from build123d import *

# Parameters (mm, degrees)
TOP_COVER_W         = 120
TOP_COVER_H         = 25
BOSS_EXTRUDE1_DEPTH = 3
ATTACHMENT_POINT_W  = 8
ATTACHMENT_POINT_H  = 15
CUT_EXTRUDE1_DEPTH  = 2
SKETCH4_R           = 1.75
M3_SCREW_CUT_DEPTH  = 62.361632964
FILLET1_R           = 2
FILLET2_R           = 2
FILLET3_R           = 2
FILLET4_R           = 2


with BuildPart() as part:
    # Top Cover → Boss-Extrude1 (new body)
    with BuildSketch(Plane(origin=(0, 0, 0), x_dir=(1, 0, 0), z_dir=(0, 1, 0))):
        Rectangle(TOP_COVER_W, TOP_COVER_H)
    extrude(amount=BOSS_EXTRUDE1_DEPTH)

    # Attachment Point → Cut-Extrude1 (cut)
    with BuildSketch(Plane(origin=(0, 3, 0), x_dir=(1, 0, 0), z_dir=(0, 1, 0))):
        with Locations((-11, 0)):
            Rectangle(ATTACHMENT_POINT_W, ATTACHMENT_POINT_H)
        with Locations((11, 0)):
            Rectangle(ATTACHMENT_POINT_W, ATTACHMENT_POINT_H)
    extrude(amount=-CUT_EXTRUDE1_DEPTH, mode=Mode.SUBTRACT)

    # Sketch4 → M3 Screw CUT (cut, through all)
    with BuildSketch(Plane(origin=(0, 3, 0), x_dir=(1, 0, 0), z_dir=(0, 1, 0))):
        with Locations(Location((-11, 0, 0), (0, 0, 270))):
            Circle(SKETCH4_R)
        with Locations(Location((11, 0, 0), (0, 0, 90))):
            Circle(SKETCH4_R)
    extrude(amount=-M3_SCREW_CUT_DEPTH, mode=Mode.SUBTRACT)

    # Fillet1
    fillet1_edges = [part.edges().sort_by_distance(p)[0] for p in [
        (-60, 1.5, 12.5),
    ]]
    fillet(fillet1_edges, radius=FILLET1_R)

    # Fillet2
    fillet2_edges = [part.edges().sort_by_distance(p)[0] for p in [
        (60, 1.5, 12.5),
    ]]
    fillet(fillet2_edges, radius=FILLET2_R)

    # Fillet3
    fillet3_edges = [part.edges().sort_by_distance(p)[0] for p in [
        (60, 1.5, -12.5),
    ]]
    fillet(fillet3_edges, radius=FILLET3_R)

    # Fillet4
    fillet4_edges = [part.edges().sort_by_distance(p)[0] for p in [
        (-60, 1.5, -12.5),
    ]]
    fillet(fillet4_edges, radius=FILLET4_R)


solid = part.part
Read the model definition and answer for the solid it produces. Units are mm, in the model's axes. A direction names the side the tool comes from. Coordinates: 2 decimals unless noted, no trailing zeros. Order: outer loops, then holes, each group sorted by start corner. A loop starts at its lowest first (then second) coordinate and runs counter-clockwise, first axis right, second up. Notation, with made-up numbers: (8, 65.5) -> (46, 65.5) arc R20 cw to (46, 100.5) -> close; hole circle Ø3 at (72.25, 30). An arc over 180 degrees is marked (long way). Answer as a JSON object with one key per item and string values.
1) A cutting plane is placed at D-D, the plane z = 5.75. Determine the outline of the cut face in (x, y).
Model answer:
{"outline": "(-60, 0) -> (60, 0) -> (60, 3) -> (15, 3) -> (15, 1) -> (7, 1) -> (7, 3) -> (-7, 3) -> (-7, 1) -> (-15, 1) -> (-15, 3) -> (-60, 3) -> close"}
2) Each of these flat-tipped pins is pushed along its axis until it touches: pin 1 (3 mm diameter, centred on x = 11, z = 0, fed in from -Y); pin 2 (3 mm diameter, centred on x = 9.5, z = 4, fed in from +Y). Where does it stop, or does it pass through?
Model answer:
{"pin 1": "passes through", "pin 2": "stops at y = 1"}
3) A cutting plane is placed at A-A, the plane x = 11. Determine the outline of the cut face in (y, z).
Model answer:
{"outline": "(0, -12.5) -> (3, -12.5) -> (3, -7.5) -> (1, -7.5) -> (1, -1.75) -> (0, -1.75) -> close; (0, 1.75) -> (1, 1.75) -> (1, 7.5) -> (3, 7.5) -> (3, 12.5) -> (0, 12.5) -> close"}
4) A cutting plane is placed at C-C, the plane y = 2. Determine the outline of the cut face in (x, z), plus the area to 3 significant figures.
Model answer:
{"outline": "(-60, -10.5) arc R2 ccw to (-58, -12.5) -> (58, -12.5) arc R2 ccw to (60, -10.5) -> (60, 10.5) arc R2 ccw to (58, 12.5) -> (-58, 12.5) arc R2 ccw to (-60, 10.5) -> close; hole (-15, -7.5) -> (-7, -7.5) -> (-7, 7.5) -> (-15, 7.5) -> close; hole (7, -7.5) -> (15, -7.5) -> (15, 7.5) -> (7, 7.5) -> close", "area": "2,760 mm²"}
5) A cutting plane is placed at B-B, the plane z = 0. Determine the outline of the cut face in (x, y).
Model answer:
{"outline": "(-60, 0) -> (-12.75, 0) -> (-12.75, 1) -> (-15, 1) -> (-15, 3) -> (-60, 3) -> close; (-9.25, 0) -> (9.25, 0) -> (9.25, 1) -> (7, 1) -> (7, 3) -> (-7, 3) -> (-7, 1) -> (-9.25, 1) -> close; (12.75, 0) -> (60, 0) -> (60, 3) -> (15, 3) -> (15, 1) -> (12.75, 1) -> close"}
6) The mould has two halves that part along X. Classify faces 1 (the face through (-60, 1, 0)), 2 (the face through (-9.265, 0.507, -0.228)), 3 (the face through (-1, 1, -12.5)): released by +X, released by -X, zero draft, split by the parting line, or undercut.
Model answer:
{"face 1": "released by -X", "face 2": "undercut", "face 3": "zero draft"}
7) A tool of negligible diameter and unlimited length cuts with its end or side. For faces 4 (the face through (59.4, 1.52, 11.93)), 5 (the face through (-11, 1, -2)), from which of +Z, -Z, +X, -X, +Y, -Y can it reach the whole face along a straight path? Write none if from no direction.
Model answer:
{"face 4": "+Z, +X, +Y, -Y", "face 5": "+Y"}
8) Consider line 1 along X through (y, z) = (2.25, -6.5); line 2 along X through (y, z) = (0.7, 0); line 3 along Z through (x, y) = (11, 0.35). Determine where each line is inside the solid, lowest interval first. Write a range as from..to.
Model answer:
{"line 1": "x = -60..-15, -7..7, 15..60", "line 2": "x = -60..-12.75, -9.25..9.25, 12.75..60", "line 3": "z = -12.5..-1.75, 1.75..12.5"}
